from build123d import *

# Parameters (mm, degrees)
SKETCH1_W                = 15.9
SKETCH1_H                = 12.7
BOSS_EXTRUDE1_DEPTH      = 1
SKETCH2_R                = 1.5
BOSS_EXTRUDE2_DEPTH      = 1
SKETCH3_W                = 15.6
SKETCH3_H                = 2.7
BOSS_EXTRUDE3_DEPTH      = 2.3
CHAMFER1_SIZE            = 0.5
SKETCH4_W                = 0.7
SKETCH4_H                = 1
BOSS_EXTRUDE4_DEPTH      = 5.9
BOSS_EXTRUDE4_DEPTH_BACK = 6
CHAMFER2_SIZE            = 0.2
CHAMFER3_SIZE            = 0.4
SKETCH5_R                = 1.8
SKETCH5_R_2              = 1.5
SKETCH5_R_3              = 0.5
BOSS_EXTRUDE5_DEPTH      = 0.0001


with BuildPart() as part:
    # Sketch1 → Boss-Extrude1 (new body, symmetric)
    with BuildSketch(Plane.XY):
        Rectangle(SKETCH1_W, SKETCH1_H)
    extrude(amount=BOSS_EXTRUDE1_DEPTH, both=True)

    # Sketch2 → Boss-Extrude2 (add, symmetric)
    with BuildSketch(Plane.XY):
        with BuildLine():
            Line((-9.75, 2.75), (-7.95, 2.75))
            Line((-7.95, 2.75), (-7.95, -2.75))
            Line((-7.95, -2.75), (-9.75, -2.75))
            ThreePointArc((-9.75, -2.75), (-12.5, 0), (-9.75, 2.75))
        make_face()
        with Locations((-9.75, 0)):
            Circle(SKETCH2_R, mode=Mode.SUBTRACT)
        with BuildLine():
            Line((9.75, -2.75), (7.95, -2.75))
            Line((7.95, -2.75), (7.95, 2.75))
            Line((7.95, 2.75), (9.75, 2.75))
            ThreePointArc((9.75, 2.75), (12.5, 0), (9.75, -2.75))
        make_face()
        with Locations((9.75, 0)):
            Circle(SKETCH2_R, mode=Mode.SUBTRACT)
    extrude(amount=BOSS_EXTRUDE2_DEPTH, both=True)

    # Sketch3 → Boss-Extrude3 (add)
    with BuildSketch(Plane(origin=(0, 0, -1), x_dir=(-1, 0, 0), z_dir=(0, 0, -1))):
        with Locations((0, -4.85)):
            Rectangle(SKETCH3_W, SKETCH3_H)
    extrude(amount=BOSS_EXTRUDE3_DEPTH)

    # Chamfer1
    chamfer1_edges = [part.edges().sort_by_distance(p)[0] for p in [
        (7.8, -3.5, -2.15),
        (7.8, -6.2, -2.15),
        (-7.8, -6.2, -2.15),
        (-7.8, -3.5, -2.15),
    ]]
    chamfer(chamfer1_edges, length=CHAMFER1_SIZE)

    # Sketch4 → Boss-Extrude4 (add, two sides)
    with BuildSketch(Plane(origin=(0, 0, -3.3), x_dir=(-1, 0, 0), z_dir=(0, 0, -1))) as boss_extrude4_sk:
        with Locations((-3.732, -4.85)):
            Rectangle(SKETCH4_W, SKETCH4_H)
        with Locations((-6.22, -4.85)):
            Rectangle(SKETCH4_W, SKETCH4_H)
        with Locations((-1.244, -4.85)):
            Rectangle(SKETCH4_W, SKETCH4_H)
        with Locations((1.244, -4.85)):
            Rectangle(SKETCH4_W, SKETCH4_H)
        with Locations((3.732, -4.85)):
            Rectangle(SKETCH4_W, SKETCH4_H)
        with Locations((6.22, -4.85)):
            Rectangle(SKETCH4_W, SKETCH4_H)
    extrude(amount=BOSS_EXTRUDE4_DEPTH)
    extrude(boss_extrude4_sk.sketch, amount=-BOSS_EXTRUDE4_DEPTH_BACK)

    # Chamfer2
    chamfer2_edges = [part.edges().sort_by_distance(p)[0] for p in [
        (4.082, -4.85, 2.7),
        (3.732, -4.35, 2.7),
        (3.382, -4.85, 2.7),
        (3.732, -5.35, 2.7),
        (4.082, -4.85, -9.2),
        (3.732, -5.35, -9.2),
        (3.382, -4.85, -9.2),
        (3.732, -4.35, -9.2),
        (1.594, -4.85, 2.7),
        (1.244, -4.35, 2.7),
        (0.894, -4.85, 2.7),
        (1.244, -5.35, 2.7),
        (1.594, -4.85, -9.2),
        (1.244, -5.35, -9.2),
        (0.894, -4.85, -9.2),
        (1.244, -4.35, -9.2),
        (-0.894, -4.85, 2.7),
        (-1.244, -4.35, 2.7),
        (-1.594, -4.85, 2.7),
        (-1.244, -5.35, 2.7),
        (-0.894, -4.85, -9.2),
        (-1.244, -5.35, -9.2),
        (-1.594, -4.85, -9.2),
        (-1.244, -4.35, -9.2),
        (-3.382, -4.85, 2.7),
        (-3.732, -4.35, 2.7),
        (-4.082, -4.85, 2.7),
        (-3.732, -5.35, 2.7),
        (-3.382, -4.85, -9.2),
        (-3.732, -5.35, -9.2),
        (-4.082, -4.85, -9.2),
        (-3.732, -4.35, -9.2),
        (-5.87, -4.85, 2.7),
        (-6.22, -4.35, 2.7),
        (-6.57, -4.85, 2.7),
        (-6.22, -5.35, 2.7),
        (-5.87, -4.85, -9.2),
        (-6.22, -5.35, -9.2),
        (-6.57, -4.85, -9.2),
        (-6.22, -4.35, -9.2),
        (6.57, -4.85, 2.7),
        (6.22, -4.35, 2.7),
        (5.87, -4.85, 2.7),
        (6.22, -5.35, 2.7),
        (6.57, -4.85, -9.2),
        (6.22, -5.35, -9.2),
        (5.87, -4.85, -9.2),
        (6.22, -4.35, -9.2),
    ]]
    chamfer(chamfer2_edges, length=CHAMFER2_SIZE)

    # Chamfer3
    chamfer3_edges = [part.edges().sort_by_distance(p)[0] for p in [
        (4.082, -4.85, 1),
        (3.732, -4.35, 1),
        (3.382, -4.85, 1),
        (3.732, -5.35, 1),
        (1.594, -4.85, 1),
        (1.244, -4.35, 1),
        (0.894, -4.85, 1),
        (1.244, -5.35, 1),
        (-0.894, -4.85, 1),
        (-1.244, -4.35, 1),
        (-1.594, -4.85, 1),
        (-1.244, -5.35, 1),
        (-3.382, -4.85, 1),
        (-3.732, -4.35, 1),
        (-4.082, -4.85, 1),
        (-3.732, -5.35, 1),
        (-5.87, -4.85, 1),
        (-6.22, -4.35, 1),
        (-6.57, -4.85, 1),
        (-6.22, -5.35, 1),
        (6.57, -4.85, 1),
        (6.22, -4.35, 1),
        (5.87, -4.85, 1),
        (6.22, -5.35, 1),
    ]]
    chamfer(chamfer3_edges, length=CHAMFER3_SIZE)

    # Sketch5 → Boss-Extrude5 (add)
    with BuildSketch(Plane.XY.offset(1)):
        with Locations((-9.75, 0)):
            Circle(SKETCH5_R)
        with Locations((-9.75, 0)):
            Circle(SKETCH5_R_2, mode=Mode.SUBTRACT)
        with Locations((9.75, 0)):
            Circle(SKETCH5_R)
        with Locations((9.75, 0)):
            Circle(SKETCH5_R_2, mode=Mode.SUBTRACT)
        with Locations((6.45, 5.1)):
            Circle(SKETCH5_R_3)
    extrude(amount=BOSS_EXTRUDE5_DEPTH)


solid = part.part
Check sheet for the modelled part. Datum: model origin and axes. Units: mm. A direction names the side the tool comes from. Round coordinates to 2 decimals unless told otherwise and drop trailing zeros. Order: outer loops, then holes, each group sorted by start corner. A loop starts at its lowest first (then second) coordinate and runs counter-clockwise, first axis right, second up.
(1) Cross-section at C-C, the plane z = -0.75. Enter the section's corners in (x, y).
(2) Cross-section at D-D, the plane z = -2. Enter the section's corners in (x, y), and give its area (3 significant figures).
(3) Scan lines: probe 1 along Y at (x, z) = (-9.75, -0.25); probe 2 along Z at (x, y) = (2.25, 2.75). Record each from-to range of solid material in increasing order.
(4) Cross-section at B-B, the plane y = 0.5. State how many separate pieces and enclosed holes the cut face has, and give its area (3 significant figures).
(5) Cross-section at A-A, the plane z = -5. Enter the section's corners in (x, y).
(6) Go/stop test with flat-tipped pins: P1, Ø0.6, axis at x = 4, z = 2, coming from the -Y side; P2, Ø0.5, axis at y = -5, z = -5, coming from the -X side; P3, Ø0.5, axis at x = -9, z = -0.5, coming from the +Y side. Record where each tip stops, or that it passes through.
(7) Draft check along X on faces 4 (the flat face through (5.87, -5, -6)), 5 (the flat face through (6.4, 5.1, 1)), 6 (the flat face through (6.57, -5, 2)). Enter one of: pulls with the +X half, pulls with the -X half, needs draft (parallel to the pull), parting line crosses it, or undercut.
(8) Access from +Z, -Z, +X, -X, +Y, -Y to the whole of each face (thin tool, end or side, straight path). Record for faces 1 (the flat face through (-7.95, 5, 0)), 2 (the flat face through (0, -3.5, -2)), 3 (the flat face through (4.082, -5, -6)).
Check sheet entries:
1. outline: (-9.75, -2.75) - (-7.95, -2.75) - (-7.95, -6.35) - (7.95, -6.35) - (7.95, -2.75) - (9.75, -2.75) arc R2.75 ccw to (9.75, 2.75) - (7.95, 2.75) - (7.95, 6.35) - (-7.95, 6.35) - (-7.95, 2.75) - (-9.75, 2.75) arc R2.75 ccw to start; hole circle Ø3 at (-9.75, 0); hole circle Ø3 at (9.75, 0)
2. outline: (-7.8, -5.7) - (-7.3, -6.2) - (7.3, -6.2) - (7.8, -5.7) - (7.8, -4) - (7.3, -3.5) - (-7.3, -3.5) - (-7.8, -4) - close
2. area: 41.6 mm2
3. probe 1: y = -2.75 to -1.5, 1.5 to 2.75
3. probe 2: z = -1 to 1
4. separate pieces: 3
4. enclosed holes: 0
4. area: 38.5 mm2
5. outline: (-6.57, -5.35) - (-5.87, -5.35) - (-5.87, -4.35) - (-6.57, -4.35) - close; (-4.08, -5.35) - (-3.38, -5.35) - (-3.38, -4.35) - (-4.08, -4.35) - close; (-1.59, -5.35) - (-0.89, -5.35) - (-0.89, -4.35) - (-1.59, -4.35) - close; (0.89, -5.35) - (1.59, -5.35) - (1.59, -4.35) - (0.89, -4.35) - close; (3.38, -5.35) - (4.08, -5.35) - (4.08, -4.35) - (3.38, -4.35) - close; (5.87, -5.35) - (6.57, -5.35) - (6.57, -4.35) - (5.87, -4.35) - close
6. P1: stops at y = -5.35
6. P2: stops at x = -6.57
6. P3: stops at y = 2.75
7. face 4: undercut
7. face 5: needs draft
7. face 6: pulls with the +X half
8. face 1: +Z, -Z, -X, +Y
8. face 2: -Z, +X, -X, +Y
8. face 3: -Z, +Y, -Y
